```python
from build123d import *

# Parameters (mm, degrees)
F0_W     = 812.8
F0_H     = 584.2
F1_DEPTH = 304.8
F2_W     = 812.8
F2_H     = 298.45
F3_DEPTH = 31.75
F4_W     = 812.8
F4_H     = 298.45
F5_DEPTH = 76.2
F6_W     = 476.25
F6_H     = 298.45
F7_DEPTH = 31.75
F8_W     = 476.25
F8_H     = 298.45
F9_DEPTH = 31.75


with BuildPart() as f1:
    # F0 (on Top) → F1 (new body)
    with BuildSketch(Plane.XY):
        Rectangle(F0_W, F0_H)
    extrude(amount=F1_DEPTH)

    # F2 (on face) → F3 (cut)
    with BuildSketch(Plane.XZ.offset(292.1)):
        with Locations((0, 149.225)):
            Rectangle(F2_W, F2_H)
    extrude(amount=-F3_DEPTH, mode=Mode.SUBTRACT)

    # F4 (on face) → F5 (cut)
    with BuildSketch(Plane(origin=(0, 292.1, 0), x_dir=(-1, 0, 0), z_dir=(0, 1, 0))):
        with Locations((0, 149.225)):
            Rectangle(F4_W, F4_H)
    extrude(amount=-F5_DEPTH, mode=Mode.SUBTRACT)

    # F6 (on face) → F7 (cut)
    with BuildSketch(Plane.YZ.offset(406.4)):
        with Locations((-22.225, 149.225)):
            Rectangle(F6_W, F6_H)
    extrude(amount=-F7_DEPTH, mode=Mode.SUBTRACT)

    # F8 (on face) → F9 (cut)
    with BuildSketch(Plane(origin=(-406.4, 0, 0), x_dir=(0, -1, 0), z_dir=(-1, 0, 0))):
        with Locations((22.225, 149.225)):
            Rectangle(F8_W, F8_H)
    extrude(amount=-F9_DEPTH, mode=Mode.SUBTRACT)


solid = f1.part
```
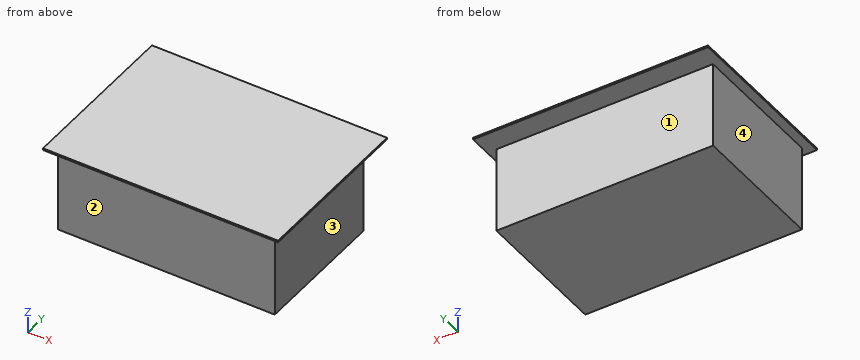
Could you check a few things on this model? Use its own coordinates, in mm. Face numbers are marked on the shaded views. A direction names the side the tool comes from. Give positions to 0.01 mm unless a question says otherwise; leave off trailing zeros. Order: outer loops, then holes, each group sorted by start corner. A loop starts at its lowest first (then second) coordinate and runs counter-clockwise, first axis right, second up.
Q1. Suppose I cut it at C-C, the plane z = 171. Write out the boundary of the cut face in (x, y), and give its area (3 significant figures).
Q2. For the marked faces 1, 2, 3 and 4, which set-ups out of +Z, -Z, +X, -X, +Y, -Y let a thin tool reach every point of the face, with its end or its side?
Q3. If I drill on line 1 along Y through (x, z) = (-53, 252.5); line 2 along X through (y, z) = (120.5, 22.5), over which ranges is the centre line in solid material (lowest first)?
Q4. Suppose I cut it at B-B, the plane y = 172. Write out the boundary of the cut face in (x, z).
Q5. I'm going to push flat-ended pins straight in: P1, Ø6, axis at y = 152, z = 137.5, coming from the +X side; P2, Ø3, axis at x = -272, y = -72, coming from the -Z side; P3, Ø1, axis at y = 111, z = 267, coming from the -X side. Where does each tip first touch, or does it pass through?
Q6. Suppose I cut it at A-A, the plane x = -176.5. Write out the boundary of the cut face in (y, z), and give its area (3 significant figures).
Solution:
1. outline: (-374.65, -260.35) - (374.65, -260.35) - (374.65, 215.9) - (-374.65, 215.9) - close
1. area: 357,000 mm2
2. face 1: -Z, +X, -X, +Y
2. face 2: -Z, +X, -X, -Y
2. face 3: -Z, +X, +Y, -Y
2. face 4: -Z, -X, +Y, -Y
3. line 1: y = -260.35 to 215.9
3. line 2: x = -374.65 to 374.65
4. outline: (-406.4, 298.45) - (-374.65, 298.45) - (-374.65, 0) - (374.65, 0) - (374.65, 298.45) - (406.4, 298.45) - (406.4, 304.8) - (-406.4, 304.8) - close
5. P1: stops at x = 374.65
5. P2: stops at z = 0
5. P3: stops at x = -374.65
6. outline: (-292.1, 298.45) - (-260.35, 298.45) - (-260.35, 0) - (215.9, 0) - (215.9, 298.45) - (292.1, 298.45) - (292.1, 304.8) - (-292.1, 304.8) - close
6. area: 146,000 mm2
